Design review of the part shown in the three views and the two pictorial views. Dimensions are in mm from the part's minimum x, y and z. Coordinates: 2 decimals unless noted, no trailing zeros. Loops run counter-clockwise (first coordinate to the right, second up) from the corner with the lowest first, then second, coordinate; pieces in that order, holes last. Notation, with made-up numbers: M -27,-18 L -10,-18 A31 ccw -10,11 Z; hole C 40,18 d2. An arc over 180 degrees is marked long. Use one line per item in the form item = value.
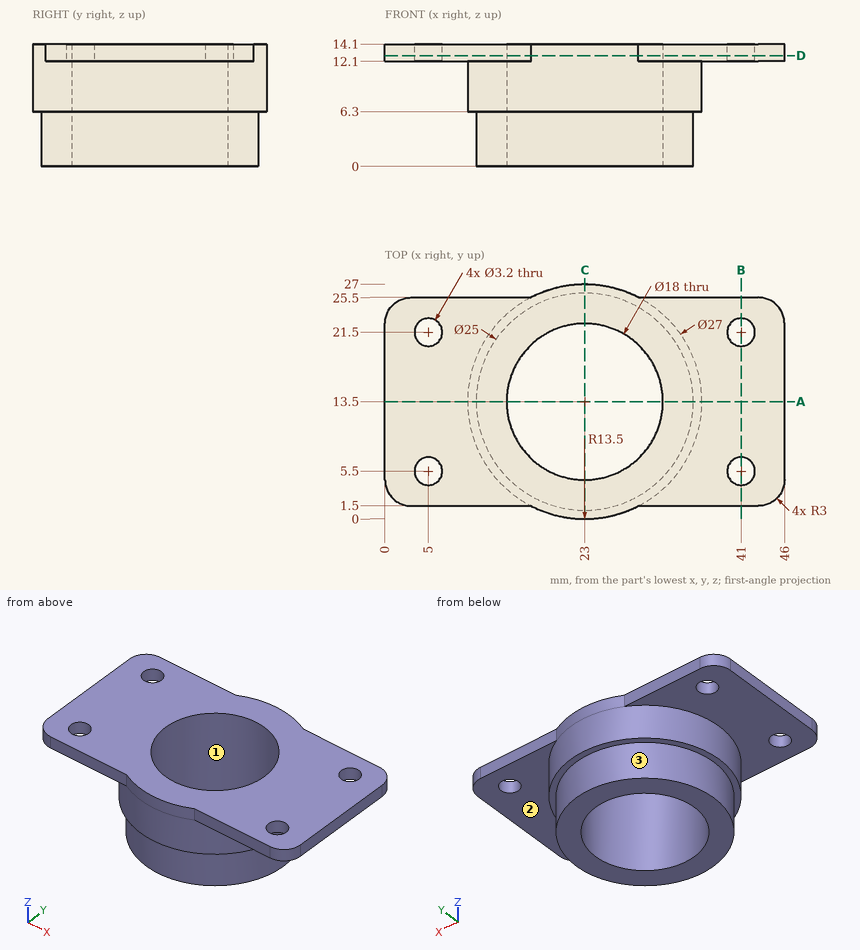
1. The part is to be moulded in two halves that separate along X. For the marked faces 1, 2 and 3, say which applies: pulls with the +X half, pulls with the -X half, needs draft (parallel to the pull), parting line crosses it, or undercut.
Response values:
face_1 = undercut
face_2 = needs draft
face_3 = parting line crosses it
2. Add section A-A (y = 13.5). State the section outline as (x, z) points, then the cut area to 3 significant figures.
Response values:
outline = M 0,12.1 L 9.5,12.1 L 9.5,6.3 L 10.5,6.3 L 10.5,0 L 14,0 L 14,14.1 L 0,14.1 Z; M 32,0 L 35.5,0 L 35.5,6.3 L 36.5,6.3 L 36.5,12.1 L 46,12.1 L 46,14.1 L 32,14.1 Z
area = 152 mm^2
3. Insertion check: P1, Ø2, axis at x = 36, z = 13.5, coming from the -Y side; P2, Ø8, axis at x = 27.5, z = 7.5, coming from the +Y side; P3, Ø4, axis at x = 41, y = 21.5, coming from the -Z side. Each pin has a flat end and moves straight along its axis. Give the tip position at first contact, or say it passes through.
Response values:
P1 = 1.5
P2 = 26.99
P3 = 12.1
4. Add section B-B (x = 41). State the section outline as (y, z) points.
Response values:
outline = M 1.5,12.1 L 3.9,12.1 L 3.9,14.1 L 1.5,14.1 Z; M 7.1,12.1 L 19.9,12.1 L 19.9,14.1 L 7.1,14.1 Z; M 23.1,12.1 L 25.5,12.1 L 25.5,14.1 L 23.1,14.1 Z
5. Add section C-C (x = 23). State the section outline as (y, z) points.
Response values:
outline = M 0,6.3 L 1,6.3 L 1,0 L 4.5,0 L 4.5,14.1 L 0,14.1 Z; M 22.5,0 L 26,0 L 26,6.3 L 27,6.3 L 27,14.1 L 22.5,14.1 Z
6. Add section D-D (z = 12.75). State the section outline as (x, y) points.
Response values:
outline = M 0,4.5 A3 ccw 3,1.5 L 16.82,1.5 A13.5 ccw 29.18,1.5 L 43,1.5 A3 ccw 46,4.5 L 46,22.5 A3 ccw 43,25.5 L 29.18,25.5 A13.5 ccw 16.82,25.5 L 3,25.5 A3 ccw 0,22.5 Z; hole C 5,5.5 d3.2; hole C 5,21.5 d3.2; hole C 23,13.5 d18; hole C 41,5.5 d3.2; hole C 41,21.5 d3.2
7. Wall thickness on line 1 along Y through (x, z) = (41, 12.9); line 2 along X through (y, z) = (13.75, 11.5); line 3 along Y through (x, z) = (23, 4.5): over which ranges is each line inside the solid? List them lowest first. Write a range as from..to.
Response values:
line_1 = 1.5..3.9, 7.1..19.9, 23.1..25.5
line_2 = 9.5..14, 32..36.5
line_3 = 1..4.5, 22.5..26
